Design review of the part built by this model. Coordinates are the model's own, in mm. A direction names the side the tool comes from. Coordinates: 2 decimals unless noted, no trailing zeros. Loops run counter-clockwise (first coordinate to the right, second up) from the corner with the lowest first, then second, coordinate; pieces in that order, holes last. Notation, with made-up numbers: (-33.75, 85) -> (-1.75, 85) arc R27 cw to (-1.75, 116) -> close; hole circle Ø4 at (89, 41.5). An arc over 180 degrees is marked (long way). Answer as a JSON object with one key per item and string values.
```python
from build123d import *

# Parameters (mm, degrees)
F1_DEPTH = 2.5
F2_DEPTH = 20
F3_D     = 5
F3_DEPTH = 200
F3_TIP   = 1.5021515476


# Not quite as in the source:
# - a feature names something its author has since deleted; it is built from what else it names


with BuildPart() as f1:
    # F0 (on Top) → F1 (new body)
    with BuildSketch(Plane.XY):
        with BuildLine():
            ThreePointArc((120.5299497215, -60.8073286712), (131.3326753181, -31.252654188), (135, 0))
            ThreePointArc((135, 0), (131.3326753181, 31.252654188), (120.5299497215, 60.8073286712))
            ThreePointArc((120.5299497215, 60.8073286712), (0, 135), (-120.5299497215, 60.8073286712))
            ThreePointArc((-120.5299497215, 60.8073286712), (-135, 0), (-120.5299497215, -60.8073286712))
            ThreePointArc((-120.5299497215, -60.8073286712), (0, -135), (120.5299497215, -60.8073286712))
        make_face()
        Polygon((88.5368213058, -73.284752667), (55.893484503, -100.0614613295), (46.9403453171, -59.9641390145), align=None, mode=Mode.SUBTRACT)
        Polygon((-117.2483563423, -17.961492762), (-117.2483563423, 31.1308540404), (-85.331723094, 0), align=None, mode=Mode.SUBTRACT)
        Polygon((58.2080259919, 55.2336238325), (72.7635622025, 97.6980701089), (103.1368598342, 61.4694543183), align=None, mode=Mode.SUBTRACT)
        with BuildLine():
            ThreePointArc((-120.5299497215, -60.8073286712), (-135, 0), (-120.5299497215, 60.8073286712))
            Line((-120.5299497215, 60.8073286712), (-167.2347635031, 60.8073286712))
            Line((-167.2347635031, 60.8073286712), (-167.2347635031, -60.8073286712))
            Line((-167.2347635031, -60.8073286712), (-120.5299497215, -60.8073286712))
        make_face()
        with BuildLine():
            ThreePointArc((120.5299497215, 60.8073286712), (131.3326753181, 31.252654188), (135, 0))
            ThreePointArc((135, 0), (131.3326753181, -31.252654188), (120.5299497215, -60.8073286712))
            Line((120.5299497215, -60.8073286712), (167.2347635031, -60.8073286712))
            Line((167.2347635031, -60.8073286712), (167.2347635031, 60.8073286712))
            Line((167.2347635031, 60.8073286712), (120.5299497215, 60.8073286712))
        make_face()
        Polygon((-85.331723094, 0), (-117.2483563423, 31.1308540404), (-117.2483563423, -17.961492762), align=None)
        Polygon((103.1368598342, 61.4694543183), (72.7635622025, 97.6980701089), (58.2080259919, 55.2336238325), align=None)
        Polygon((46.9403453171, -59.9641390145), (55.893484503, -100.0614613295), (88.5368213058, -73.284752667), align=None)
    extrude(amount=F1_DEPTH)

    # F0 (on Top) → F2 (join)
    with BuildSketch(Plane.XY):
        Polygon((-85.331723094, 0), (-117.2483563423, 31.1308540404), (-117.2483563423, -17.961492762), align=None)
        Polygon((103.1368598342, 61.4694543183), (72.7635622025, 97.6980701089), (58.2080259919, 55.2336238325), align=None)
        Polygon((46.9403453171, -59.9641390145), (55.893484503, -100.0614613295), (88.5368213058, -73.284752667), align=None)
    extrude(amount=-F2_DEPTH)

    # F3
    with Locations(Plane(origin=(0, 0, 0), x_dir=(1, 0, 0), z_dir=(0, 0, -1))):
        with Locations((-40.2909182012, -57.7073432505), (-40.2909182012, -38.0536355078), (-40.2909182012, -9.2816902325), (-40.2909182012, 8.147473447), (-40.2909182012, 49.0921735764), (-30.054744333, 33.8762365282), (-16.7753826827, 49.0921735764), (-20.6485316157, 19.2136075348), (-20.6485316157, 0), (-20.6485316157, -19.7945162654), (-16.7753826827, -38.0536355078), (-26.1815954, -52.7162663639), (0, -53.5462275147), (11.7199122906, -38.0536355078), (0, -19.7945162654), (0, 19.2136075348), (0, 36.0894650221), (13.9331379905, 49.0921735764), (42.1517826617, 49.0921735764), (32.7455736697, 33.0462753773), (21.4027836919, 19.2136075348), (21.4027836919, 0), (21.4027836919, -19.7945162654), (29.7023877501, -51.8863089383), (42.1517826617, -58.9785054326), (42.1517826617, -38.0536355078), (42.1517826617, -9.2816902325), (42.1517826617, 10.3607000783)):
            Hole(F3_D / 2, depth=F3_DEPTH)
            with Locations((0, 0, -(F3_DEPTH + F3_TIP / 2))):  # 118° drill point
                Cone(0, F3_D / 2, F3_TIP, mode=Mode.SUBTRACT)


solid = f1.part
```
1) Add section C-C, the plane x = 51.5. Give the boundary of the cut face in (y, z), and give its area (3 significant figures).
Completed:
{"outline": "(-124.79, 0) -> (-80.38, 0) -> (-80.38, -20) -> (-61.42, -20) -> (-61.42, 0) -> (124.79, 0) -> (124.79, 2.5) -> (-124.79, 2.5) -> close", "area": "1,000 mm²"}
2) Wall thickness on probe 1 along Y at (x, z) = (0, 1.45); probe 2 along Z at (x, y) = (-67, -66.5); probe 3 along X at (y, z) = (76, -14): over which ranges is each line inside the solid? List them lowest first.
Completed:
{"probe 1": "-135 to -38.59, -33.59 to -21.71, -16.71 to 17.29, 22.29 to 51.05, 56.05 to 135", "probe 2": "0 to 2.5", "probe 3": "65.33 to 90.95"}
3) The part is to be moulded in two halves that separate along Y. For faces 1 (the cylindrical face through (-2.086, -134.984, 1.232)), 2 (the flat face through (-101.07, 15.35, -9.86)), 3 (the flat face through (80.36, 58.31, -9.86)), say which applies: pulls with the +Y half, pulls with the -Y half, needs draft (parallel to the pull), parting line crosses it, or undercut.
Completed:
{"face 1": "pulls with the -Y half", "face 2": "pulls with the +Y half", "face 3": "undercut"}
4) Clearance check with flat-ended pins moving along their axes: pin 1 Ø6 at (x, y) = (-30.05, -33.88) entering from -Z; pin 2 Ø12 at (x, z) = (-93, -1.5) entering from +Y; pin 3 Ø5 at (y, z) = (-77.5, -6.5) entering from -X. State where each tip first meets the part, or that it passes through.
Completed:
{"pin 1": "z = 0", "pin 2": "y = 103.07", "pin 3": "x = 50.3"}
5) Add section A-A, the plane z = -10.75. Give the boundary of the cut face in (x, y), and give its area (3 significant figures).
Completed:
{"outline": "(-117.25, -17.96) -> (-85.33, 0) -> (-117.25, 31.13) -> close; (46.94, -59.96) -> (55.89, -100.06) -> (88.54, -73.28) -> close; (58.21, 55.23) -> (103.14, 61.47) -> (72.76, 97.7) -> close", "area": "2,470 mm²"}
6) Add section D-D, the plane x = -128. Give the boundary of the cut face in (y, z), and give its area (3 significant figures).
Completed:
{"outline": "(-60.81, 0) -> (60.81, 0) -> (60.81, 2.5) -> (-60.81, 2.5) -> close", "area": "304 mm²"}
7) Add section B-B, the plane y = -88. Give the boundary of the cut face in (x, z).
Completed:
{"outline": "(-102.38, 0) -> (53.2, 0) -> (53.2, -20) -> (70.6, -20) -> (70.6, 0) -> (102.38, 0) -> (102.38, 2.5) -> (-102.38, 2.5) -> close"}
8) For faces 4 (the flat face through (68.03, -66.718, -9.86)), 5 (the flat face through (88.163, 79.33, -9.86)), 6 (the flat face through (-117.248, 7, -10)), 7 (the flat face through (71.99, -86.86, -9.86)), 8 (the flat face through (51.354, -79.732, -9.86)), list the 3-axis set-ups (+Z, -Z, +X, -X, +Y, -Y) from which the entire face can be reached by the end or side of a thin tool; tool diameter is ignored.
Completed:
{"face 4": "-Z, +X", "face 5": "-Z, +X, +Y", "face 6": "-Z, -X, +Y, -Y", "face 7": "-Z, +X, -Y", "face 8": "-Z, -X, -Y"}
